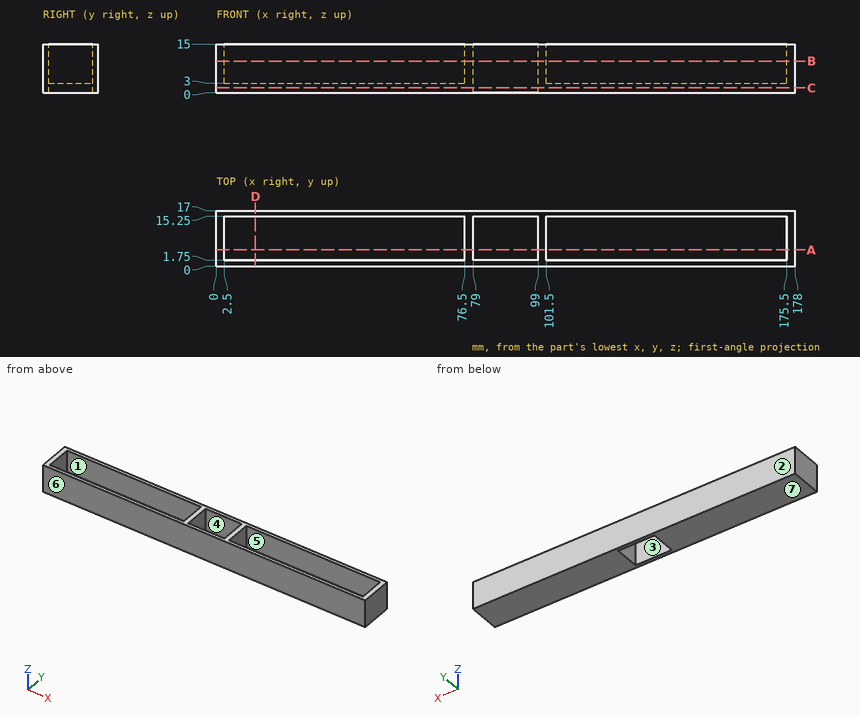
Geometry: see drawing. Coordinates: mm, zero at the bounding-box minimum. A direction names the side the tool comes from. Give positions to 0.01 mm unless a question says otherwise; leave off trailing zeros. Loops run counter-clockwise (first coordinate to the right, second up) from the corner with the lowest first, then second, coordinate; pieces in that order, holes last. Notation, with made-up numbers: (-37.75, 25) - (9.25, 25) arc R16 cw to (9.25, 36) - close; hole circle Ø2 at (60.5, -19). An arc over 180 degrees is marked (long way). Use CSV: the item, a comma, the result in double quotes. Start each with the question number.
1. Section D-D (x = 12). Output: boundary loops of the cut face in (y, z).
2. Section C-C (z = 1.5). Output: boundary loops of the cut face in (x, y).
3. Section A-A (y = 5). Output: boundary loops of the cut face in (x, z), then the cut area to 3 significant figures.
4. Reachability of the marked faces 1, 2 and 3 from +Z, -Z, +X, -X, +Y, -Y: full face, straight path, thin tool, end or side. Return the list, or none.
5. Pin query (flat end, axial travel): pin 1 (4 mm diameter, centred on x = 122, y = 8.5, fed in from +Z); pin 2 (10 mm diameter, centred on x = 57.5, y = 13, fed in from +Z). Return the tip coordinate at first contact, or that it passes through.
6. Section B-B (z = 9.75). Output: boundary loops of the cut face in (x, y).
7. Ray query, L1, parallel to X at y = 6, z = 5.5; L2, parallel to Y at x = 96, z = 1.5; L3, parallel to X at y = 11.5, z = 2.5. Return the intervals inside material, ascending.
8. Draft query along Y for the marked faces 4, 5, 6 and 7. Return one class per face: +Y half, -Y half, draft (parallel to the pull), parting line (faces both ways), or undercut.
Response:
1,outline,"(0, 0) - (17, 0) - (17, 15) - (15.25, 15) - (15.25, 3) - (1.75, 3) - (1.75, 15) - (0, 15) - close"
2,outline,"(0, 0) - (178, 0) - (178, 17) - (0, 17) - close; hole (79, 1.75) - (99, 1.75) - (99, 15.25) - (79, 15.25) - close"
3,outline,"(0, 0) - (79, 0) - (79, 15) - (76.5, 15) - (76.5, 3) - (2.5, 3) - (2.5, 15) - (0, 15) - close; (99, 0) - (178, 0) - (178, 15) - (175.5, 15) - (175.5, 3) - (101.5, 3) - (101.5, 15) - (99, 15) - close"
3,area,"594 mm²"
4,face 1,"+Z"
4,face 2,"+Z, -Z, +X, -X, +Y"
4,face 3,"+Z, -Z"
5,pin 1,"z = 3"
5,pin 2,"z = 15"
6,outline,"(0, 0) - (178, 0) - (178, 17) - (0, 17) - close; hole (2.5, 1.75) - (76.5, 1.75) - (76.5, 15.25) - (2.5, 15.25) - close; hole (79, 1.75) - (99, 1.75) - (99, 15.25) - (79, 15.25) - close; hole (101.5, 1.75) - (175.5, 1.75) - (175.5, 15.25) - (101.5, 15.25) - close"
7,L1,"0 to 2.5, 76.5 to 79, 99 to 101.5, 175.5 to 178"
7,L2,"0 to 1.75, 15.25 to 17"
7,L3,"0 to 79, 99 to 178"
8,face 4,"undercut"
8,face 5,"undercut"
8,face 6,"-Y half"
8,face 7,"draft"
